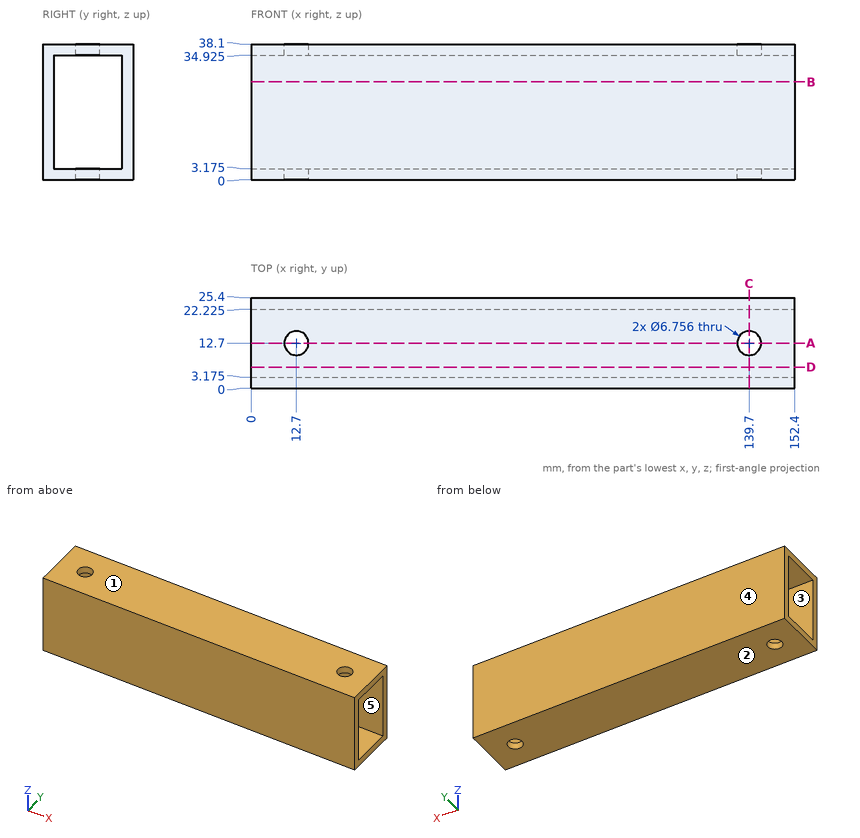
For this review, use the dimensioned drawing (mm, ordinates from the lowest corner) and the shaded views. A direction names the side the tool comes from. Round coordinates to 2 decimals unless told otherwise and drop trailing zeros. Write each loop counter-clockwise with the first axis right and the second up, starting at its lowest first coordinate (ties: lowest second). Pieces come first, ordered by that corner, then holes. Notation, with made-up numbers: (21.25, 12.25) -> (76.25, 12.25) arc R29 ccw to (76.25, 32.25) -> close; hole circle Ø9 at (-17, -13.75). An arc over 180 degrees is marked (long way). Use one line per item in the form item = value.
Q1. To check wall thickness, follow probe 1 along Z at (x, y) = (122, 18.5) (1 decimal); probe 2 along Y at (x, z) = (82, 7) (1 decimal); probe 3 along X at (y, z) = (11.5, 3). State the ranges of each line that lie inside material, in increasing order. Write a range as from..to.
Resolved:
probe_1 = 0..3.2, 34.9..38.1
probe_2 = 0..3.2, 22.2..25.4
probe_3 = 0..9.54, 15.86..136.54, 142.86..152.4
Q2. Consider section C-C (x = 139.7). State the section outline as (y, z) points (1 decimal).
Resolved:
outline = (0, 0) -> (9.3, 0) -> (9.3, 3.2) -> (3.2, 3.2) -> (3.2, 34.9) -> (9.3, 34.9) -> (9.3, 38.1) -> (0, 38.1) -> close; (16.1, 0) -> (25.4, 0) -> (25.4, 38.1) -> (16.1, 38.1) -> (16.1, 34.9) -> (22.2, 34.9) -> (22.2, 3.2) -> (16.1, 3.2) -> close
Q3. Machinability: for the marked faces 4 and 5, which of the approach directions +Z, -Z, +X, -X, +Y, -Y give a long, thin tool a straight path to every point of the face, cutting with its end or side? Answer none if there is none.
Resolved:
face_4 = +Z, -Z, +X, -X, +Y
face_5 = +X, -X
Q4. The part is to be moulded in two halves that separate along Z. For the marked faces 1, 2 and 3, say which applies: released by +Z, released by -Z, zero draft, split by the parting line, or undercut.
Resolved:
face_1 = released by +Z
face_2 = released by -Z
face_3 = undercut
Q5. Consider section D-D (y = 6). State the section outline as (x, z) points (1 decimal).
Resolved:
outline = (0, 0) -> (152.4, 0) -> (152.4, 3.2) -> (0, 3.2) -> close; (0, 34.9) -> (152.4, 34.9) -> (152.4, 38.1) -> (0, 38.1) -> close
Q6. Consider section B-B (z = 27.5). State the section outline as (x, y) points (1 decimal).
Resolved:
outline = (0, 0) -> (152.4, 0) -> (152.4, 3.2) -> (0, 3.2) -> close; (0, 22.2) -> (152.4, 22.2) -> (152.4, 25.4) -> (0, 25.4) -> close
Q7. Consider section A-A (y = 12.7). State the section outline as (x, z) points (1 decimal).
Resolved:
outline = (0, 0) -> (9.3, 0) -> (9.3, 3.2) -> (0, 3.2) -> close; (0, 34.9) -> (9.3, 34.9) -> (9.3, 38.1) -> (0, 38.1) -> close; (16.1, 0) -> (136.3, 0) -> (136.3, 3.2) -> (16.1, 3.2) -> close; (16.1, 34.9) -> (136.3, 34.9) -> (136.3, 38.1) -> (16.1, 38.1) -> close; (143.1, 0) -> (152.4, 0) -> (152.4, 3.2) -> (143.1, 3.2) -> close; (143.1, 34.9) -> (152.4, 34.9) -> (152.4, 38.1) -> (143.1, 38.1) -> close
